The drawing under review shows one solid part. Ordinate dimensions are in mm from its lowest x, y, z. Round coordinates to 2 decimals unless told otherwise and drop trailing zeros. Write each loop counter-clockwise with the first axis right and the second up, starting at its lowest first coordinate (ties: lowest second). Pieces come first, ordered by that corner, then holes. Notation, with made-up numbers: (54.5, 33) -> (62.5, 33) arc R19 ccw to (62.5, 47) -> close; hole circle Ø7 at (10.25, 87.5). An arc over 180 degrees is marked (long way). Write item = value, one per line. Start each with the question number.
Item 1: Mouldability with a two-part tool opening along X and no side actions: class the marked faces 1, 2 and 3 as released by +X, released by -X, zero draft, split by the parting line, or undercut.
Item 2: Add section C-C, the plane y = 48. State the section outline as (x, z) points, then the cut area to 3 significant figures.
Item 3: For pin 1 Ø6 at (x, y) = (45, 13.5) entering from +Z; pin 2 Ø10 at (x, z) = (89.5, 50) entering from -Y; pin 3 Ø12 at (x, y) = (80, 39.5) entering from -Z, all flat-tipped, find the tip position at first contact; note any pin that passes through.
Item 4: Add section A-A, the plane z = 50. State the section outline as (x, y) points.
Item 5: To check wall thickness, follow L1, parallel to Z at x = 50, y = 51.3; L2, parallel to Z at x = 50, y = 30; L3, parallel to Y at x = 43, z = 80. State the ranges of each line that lie inside material, in increasing order.
Item 6: Add section B-B, the plane x = 50. State the section outline as (y, z) points, then the cut area to 3 significant figures.
Item 7: Add section D-D, the plane z = 13. State the section outline as (x, y) points, then the cut area to 3 significant figures.
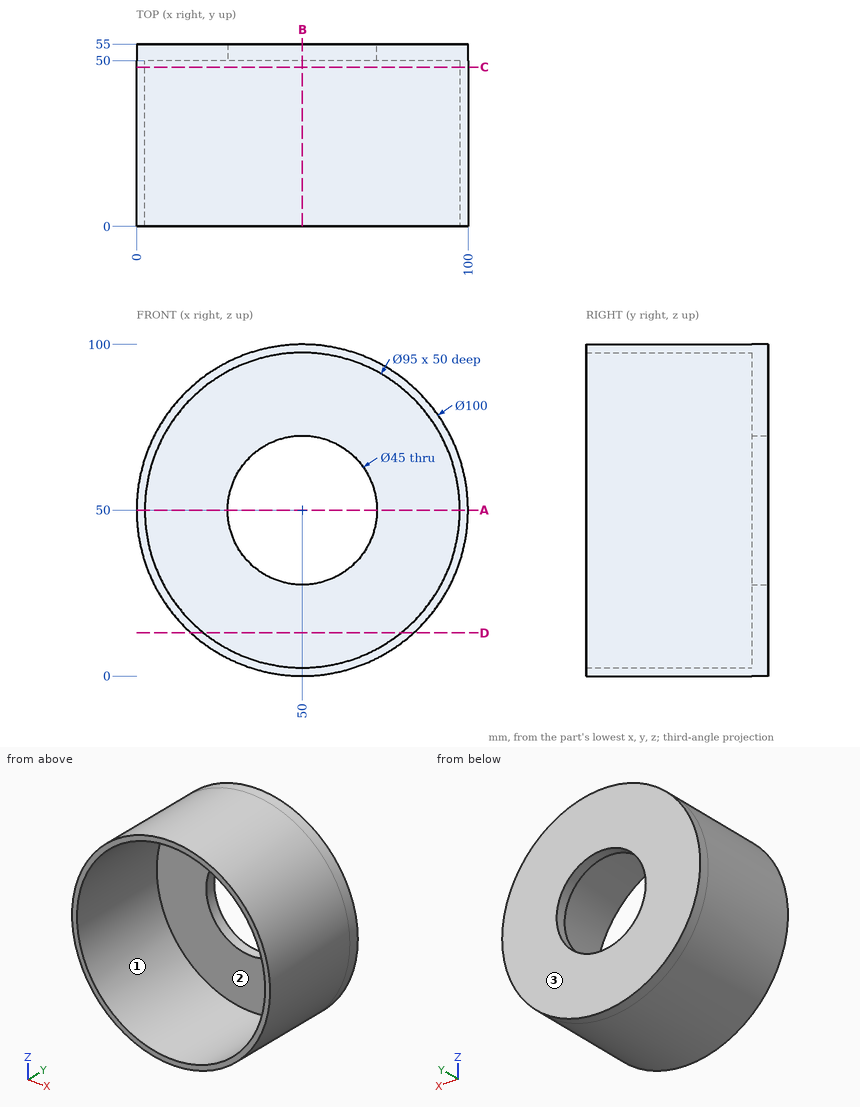
Result set:
q1.face_1 = undercut
q1.face_2 = undercut
q1.face_3 = zero draft
q2.outline = circle Ø100 at (50, 50); hole circle Ø95 at (50, 50)
q2.area = 766 mm²
q3.pin_1 = 99.96
q3.pin_2 = 50
q3.pin_3 = 6.14
q4.outline = (0, 0) -> (2.5, 0) -> (2.5, 50) -> (27.5, 50) -> (27.5, 55) -> (0, 55) -> close; (72.5, 50) -> (97.5, 50) -> (97.5, 0) -> (100, 0) -> (100, 55) -> (72.5, 55) -> close
q5.L1 = 0 to 27.5, 72.5 to 100
q5.L2 = 0 to 2.5, 97.5 to 100
q5.L3 = 50 to 55
q6.outline = (0, 0) -> (55, 0) -> (55, 27.5) -> (50, 27.5) -> (50, 2.5) -> (0, 2.5) -> close; (0, 97.5) -> (50, 97.5) -> (50, 72.5) -> (55, 72.5) -> (55, 100) -> (0, 100) -> close
q6.area = 525 mm²
q7.outline = (16.37, 0) -> (20.21, 0) -> (20.21, 50) -> (79.79, 50) -> (79.79, 0) -> (83.63, 0) -> (83.63, 55) -> (16.37, 55) -> close
q7.area = 721 mm²
